For this review, take the finished solid that the model builds, in its own axes (mm). Coordinates: 2 decimals unless noted, no trailing zeros. Order: outer loops, then holes, each group sorted by start corner. A loop starts at its lowest first (then second) coordinate and runs counter-clockwise, first axis right, second up. Notation, with made-up numbers: (53, 70) - (111, 70) arc R14 ccw to (111, 79) - close; hole circle Ø11 at (19.5, 48.5). An arc over 180 degrees is marked (long way). One line per item, written item: value. Start each with the question number.
(1) Consider section C-C on z = 2.2. Write out the cut boundary in (x, y), then the cut area to 3 significant figures.
(2) Mouldability with a two-part tool opening along Y and no side actions: class faces 1 (the cylindrical face through (-0.74, -3.32, 1.18)), 2 (the cylindrical face through (-2.084, 0.656, 2.146)), 3 (the flat face through (-2, 2, 2.4)) as released by +Y, released by -Y, zero draft, split by the parting line, or undercut.
(3) Consider section A-A on x = 0. Write out the cut boundary in (y, z), then the cut area to 3 significant figures.
(4) To check wall thickness, follow line 1 along Y through (x, z) = (0, 0.35); line 2 along X through (y, z) = (0.5, 2); line 3 along Y through (x, z) = (0, 2.1). State the ranges of each line that lie inside material, in increasing order.
(5) Consider section B-B on z = 0.25. Write out the cut boundary in (x, y).
```python
from build123d import *

# Parameters (mm, degrees)
SKETCH1_R           = 3.4
BOSS_EXTRUDE1_DEPTH = 2.4
SKETCH2_R           = 1.55
CUT_EXTRUDE1_DEPTH  = 0.8
SKETCH3_R           = 1.55
CUT_EXTRUDE2_DEPTH  = 1.1
CUT_EXTRUDE2_TAPER  = -30
CUT_EXTRUDE3_REACH  = 2.5
SKETCH4_R           = 2.185085296


with BuildPart() as part:
    # Sketch1 → Boss-Extrude1 (new body)
    with BuildSketch(Plane.XY):
        Circle(SKETCH1_R)
    extrude(amount=BOSS_EXTRUDE1_DEPTH)

    # Sketch2 → Cut-Extrude1 (cut)
    with BuildSketch(Plane(origin=(0, 0, 0), x_dir=(-1, 0, 0), z_dir=(0, 0, -1))):
        Circle(SKETCH2_R)
    extrude(amount=-CUT_EXTRUDE1_DEPTH, mode=Mode.SUBTRACT)

    # Sketch3 → Cut-Extrude2 (cut)
    with BuildSketch(Plane(origin=(0, 0, 0.8), x_dir=(-1, 0, 0), z_dir=(0, 0, -1))):
        Circle(SKETCH3_R)
    extrude(amount=-CUT_EXTRUDE2_DEPTH, taper=CUT_EXTRUDE2_TAPER, mode=Mode.SUBTRACT)

    # Sketch4 → Cut-Extrude3 (cut, up to next)
    with BuildSketch(Plane(origin=(0, 0, 1.9), x_dir=(-1, 0, 0), z_dir=(0, 0, -1)), mode=Mode.PRIVATE) as cut_extrude3_sk1:
        Circle(SKETCH4_R)
    cut_extrude3_tool1 = extrude(cut_extrude3_sk1.sketch, amount=-CUT_EXTRUDE3_REACH, mode=Mode.PRIVATE) & part.part
    add(cut_extrude3_tool1.solids().sort_by_distance((0, 0, 1.9))[0], mode=Mode.SUBTRACT)


solid = part.part
```
Geometry check:
1. outline: circle Ø6.8 at (0, 0); hole circle Ø4.37 at (0, 0)
1. area: 21.3 mm^2
2. face 1: split by the parting line
2. face 2: undercut
2. face 3: zero draft
3. outline: (-3.4, 0) - (-1.55, 0) - (-1.55, 0.8) - (-2.19, 1.9) - (-2.19, 2.4) - (-3.4, 2.4) - close; (1.55, 0) - (3.4, 0) - (3.4, 2.4) - (2.19, 2.4) - (2.19, 1.9) - (1.55, 0.8) - close
3. area: 7.55 mm^2
4. line 1: y = -3.4 to -1.55, 1.55 to 3.4
4. line 2: x = -3.36 to -2.13, 2.13 to 3.36
4. line 3: y = -3.4 to -2.19, 2.19 to 3.4
5. outline: circle Ø6.8 at (0, 0); hole circle Ø3.1 at (0, 0)
